For this review, take the finished solid that the model builds, in its own axes (mm). A direction names the side the tool comes from. Round coordinates to 2 decimals unless told otherwise and drop trailing zeros. Loops run counter-clockwise (first coordinate to the right, second up) from the corner with the lowest first, then second, coordinate; pieces in that order, holes last.
1. Consider section C-C on z = 43.5. State the section outline as (x, y) points, then the cut area to 3 significant figures.
2. Consider section A-A on z = -24. State the section outline as (x, y) points.
3. To check wall thickness, follow line 1 along X through (y, z) = (3.45, 47.5); line 2 along X through (y, z) = (2.9, -54); line 3 along Z through (x, y) = (-12.5, 0.85). State the ranges of each line that lie inside material, in increasing order.
4. Tool access review of faces 1 (the flat face through (12, 2, 54)), 2 (the flat face through (0, 0, -1)): name each direction out of +Z, -Z, +X, -X, +Y, -Y from which nothing blocks a thin tool from reaching the whole face with its end or side.
5. Consider section B-B on y = 0.85. State how many separate pieces and enclosed holes the cut face has, then the cut area to 3 significant figures.
6. Draft analysis for pull direction X (two halves, no side actions). For faces 3 (the cylindrical face through (28.58, 1.97, -68.29)), 4 (the flat face through (-13, 2, 54)), 5 (the cylindrical face through (-28.29, 1.97, -68.58)), 6 (the flat face through (14, 2, 44)), state which applies: released by +X, released by -X, zero draft, split by the parting line, or undercut.
7. Clearance check with flat-ended pins moving along their axes: pin 1 Ø3.5 at (x, z) = (27, 55) entering from -Y; pin 2 Ø2 at (x, y) = (-17.5, 2.5) entering from +Z. State where each tip first meets the part, or that it passes through.
from build123d import *

# Parameters (mm, degrees)
SKETCH1_R                                     = 3.5
SKETCH1_R_2                                   = 1.5
SKETCH1_W                                     = 3
SKETCH1_H                                     = 20
BOSS_EXTRUDE1_DEPTH                           = 4
CSK_FOR_M5_COUNTERSUNK_FLAT_HEAD1_AT_2_COUNT  = 2
CSK_FOR_M5_COUNTERSUNK_FLAT_HEAD1_AT_2_PITCH  = 110
CSK_FOR_M3_COUNTERSUNK_FLAT_HEAD1_D           = 3.4
CSK_FOR_M3_COUNTERSUNK_FLAT_HEAD1_DEPTH       = 4
CSK_FOR_M3_COUNTERSUNK_FLAT_HEAD1_CSINK_D     = 6.3
CSK_FOR_M3_COUNTERSUNK_FLAT_HEAD1_CSINK_ANGLE = 90


with BuildPart() as part:
    # Sketch1 → Boss-Extrude1 (new body)
    with BuildSketch(Plane(origin=(0, 0, 0), x_dir=(1, 0, 0), z_dir=(0, 1, 0))):
        with BuildLine():
            Line((-15, -74), (15, -74))
            ThreePointArc((15, -74), (28.435028843, -68.435028843), (34, -55))
            Line((34, -55), (34, 55))
            ThreePointArc((34, 55), (28.435028843, 68.435028843), (15, 74))
            Line((15, 74), (-15, 74))
            ThreePointArc((-15, 74), (-28.435028843, 68.435028843), (-34, 55))
            Line((-34, 55), (-34, -55))
            ThreePointArc((-34, -55), (-28.435028843, -68.435028843), (-15, -74))
        make_face()
        with Locations(Location((-15, 54, 0), (0, 0, 270))):
            Circle(SKETCH1_R, mode=Mode.SUBTRACT)
        with Locations(Location((-15, 24, 0), (0, 0, 270))):
            Circle(SKETCH1_R, mode=Mode.SUBTRACT)
        with Locations(Location((15, 24, 0), (0, 0, 270))):
            Circle(SKETCH1_R, mode=Mode.SUBTRACT)
        with Locations(Location((15, 54, 0), (0, 0, 270))):
            Circle(SKETCH1_R, mode=Mode.SUBTRACT)
        with Locations(Location((-12.5, -30, 0), (0, 0, 270))):
            Circle(SKETCH1_R_2, mode=Mode.SUBTRACT)
        with Locations(Location((-12.5, -58, 0), (0, 0, 270))):
            Circle(SKETCH1_R_2, mode=Mode.SUBTRACT)
        with Locations(Location((12.5, -30, 0), (0, 0, 90))):
            Circle(SKETCH1_R_2, mode=Mode.SUBTRACT)
        with Locations(Location((12.5, -58, 0), (0, 0, 90))):
            Circle(SKETCH1_R_2, mode=Mode.SUBTRACT)
        with Locations((-12.5, -44)):
            Rectangle(SKETCH1_W, SKETCH1_H, mode=Mode.SUBTRACT)
        with Locations((12.5, -44)):
            Rectangle(SKETCH1_W, SKETCH1_H, mode=Mode.SUBTRACT)
    extrude(amount=BOSS_EXTRUDE1_DEPTH)

    # Sketch3 → CSK for M5 Countersunk Flat Head1 (revolve, cut)
    with BuildSketch(Plane(origin=(27, 4, -55), x_dir=(0, 0, 1), z_dir=(1, 0, 0))):
        Polygon((0, 0), (0, 4), (2.75, 4), (2.75, 2.45), (5.2, 0), align=None)
    csk_for_m5_countersunk_flat_head1 = revolve(axis=Axis((27, 10.35, -55), (0, -1, 0)), mode=Mode.SUBTRACT)

    # CSK for M5 Countersunk Flat Head1 at 2: CSK for M5 Countersunk Flat Head1 ×2
    with Locations(*[(0, 0, i * CSK_FOR_M5_COUNTERSUNK_FLAT_HEAD1_AT_2_PITCH) for i in range(1, CSK_FOR_M5_COUNTERSUNK_FLAT_HEAD1_AT_2_COUNT)]):
        add(csk_for_m5_countersunk_flat_head1, mode=Mode.SUBTRACT)

    # CSK for M3 Countersunk Flat Head1
    with Locations(Plane(origin=(0, 4, 0), x_dir=(1, 0, 0), z_dir=(0, 1, 0))):
        with Locations((-12.5, -30), (12.5, -30), (12.5, -58), (-12.5, -58)):
            CounterSinkHole(CSK_FOR_M3_COUNTERSUNK_FLAT_HEAD1_D / 2, CSK_FOR_M3_COUNTERSUNK_FLAT_HEAD1_CSINK_D / 2, depth=CSK_FOR_M3_COUNTERSUNK_FLAT_HEAD1_DEPTH, counter_sink_angle=CSK_FOR_M3_COUNTERSUNK_FLAT_HEAD1_CSINK_ANGLE)


solid = part.part
Resolved:
1. outline: (-34, 0) - (-14, 0) - (-14, 4) - (-34, 4) - close; (-11, 0) - (11, 0) - (11, 4) - (-11, 4) - close; (14, 0) - (34, 0) - (34, 4) - (14, 4) - close
1. area: 248 mm2
2. outline: (-34, 0) - (-18.5, 0) - (-18.5, 4) - (-34, 4) - close; (-11.5, 0) - (11.5, 0) - (11.5, 4) - (-11.5, 4) - close; (18.5, 0) - (34, 0) - (34, 4) - (18.5, 4) - close
3. line 1: x = -34 to -14, -11 to 11, 14 to 34
3. line 2: x = -34 to -18.5, -11.5 to 11.5, 18.5 to 23.02, 30.98 to 34
3. line 3: z = -74 to -56.45, -51.55 to -26.45, -21.55 to 28.3, 31.7 to 34, 54 to 56.3, 59.7 to 74
4. face 1: +Y, -Y
4. face 2: +Z, -Z, +X, -X, -Y
5. separate pieces: 1
5. enclosed holes: 12
5. area: 9,400 mm2
6. face 3: released by +X
6. face 4: undercut
6. face 5: released by -X
6. face 6: undercut
7. pin 1: passes through
7. pin 2: stops at z = 73.94
